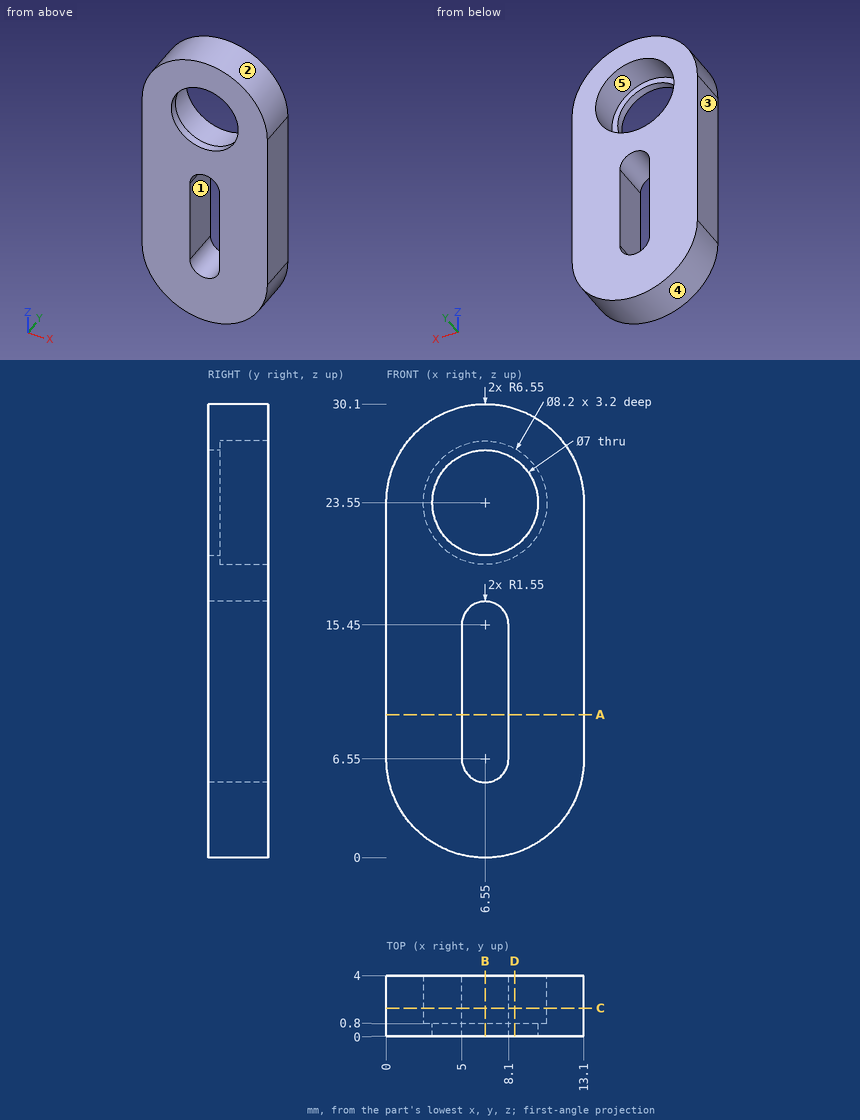
The figure shows three views and two pictorial views of one solid part (mm, origin at its lowest corner). Answer the questions. A direction names the side the tool comes from. Coordinates: 2 decimals unless noted, no trailing zeros. Loops run counter-clockwise (first coordinate to the right, second up) from the corner with the lowest first, then second, coordinate; pieces in that order, holes last. Notation, with made-up numbers: (-22, -2.75) -> (34, -2.75) arc R21 ccw to (34, 35.25) -> close; hole circle Ø3 at (15, 77.5). An arc over 180 degrees is marked (long way). Use one line per item in the form item = value. Start each with the question number.
Item 1: A tool of negligible diameter and unlimited length cuts with its end or side. For the marked faces 1 and 2, from which of +Z, -Z, +X, -X, +Y, -Y can it reach the whole face along a straight path? Write none if from no direction.
Item 2: The part is cut by section B-B on x = 6.55. Determine the outline of the cut face in (y, z), then the cut area to 3 significant figures.
Item 3: Consider L1, parallel to Z at x = 6.55, y = 2.35; L2, parallel to Z at x = 6.55, y = 0.3; L3, parallel to X at y = 3.45, z = 12.5. Determine where each line is inside the solid, lowest interval first. Write a range as [from, to].
Item 4: Flat-ended cylindrical pins translate along their axes: pin 1 Ø3 at (x, z) = (3, 9.5) entering from -Y; pin 2 Ø1 at (x, y) = (11.5, 1) entering from -Z; pin 3 Ø6.5 at (x, z) = (6.55, 23.55) entering from +Y. Find the tip coordinate at first contact, or state that the pin passes through.
Item 5: The mould has two halves that part along X. Classify the marked faces 3, 4 and 5: released by +X, released by -X, zero draft, split by the parting line, or undercut.
Item 6: The part is cut by section A-A on z = 9.5. Determine the outline of the cut face in (x, y), then the cut area to 3 significant figures.
Item 7: The part is cut by section C-C on y = 1.85. Determine the outline of the cut face in (x, z), then the cut area to 3 significant figures.
Item 8: The part is cut by section D-D on x = 8.5. Determine the outline of the cut face in (y, z), then the cut area to 3 significant figures.
Answer key:
q1.face_1 = +Y, -Y
q1.face_2 = +Z, +Y, -Y
q2.outline = (0, 0) -> (4, 0) -> (4, 5) -> (0, 5) -> close; (0, 17) -> (4, 17) -> (4, 19.45) -> (0.8, 19.45) -> (0.8, 20.05) -> (0, 20.05) -> close; (0, 27.05) -> (0.8, 27.05) -> (0.8, 27.65) -> (4, 27.65) -> (4, 30.1) -> (0, 30.1) -> close
q2.area = 40.6 mm2
q3.L1 = [0, 5], [17, 19.45], [27.65, 30.1]
q3.L2 = [0, 5], [17, 20.05], [27.05, 30.1]
q3.L3 = [0, 5], [8.1, 13.1]
q4.pin_1 = 0
q4.pin_2 = 1.74
q4.pin_3 = through
q5.face_3 = released by -X
q5.face_4 = split by the parting line
q5.face_5 = undercut
q6.outline = (0, 0) -> (5, 0) -> (5, 4) -> (0, 4) -> close; (8.1, 0) -> (13.1, 0) -> (13.1, 4) -> (8.1, 4) -> close
q6.area = 40.0 mm2
q7.outline = (0, 6.55) arc R6.55 ccw to (13.1, 6.55) -> (13.1, 23.55) arc R6.55 ccw to (0, 23.55) -> close; hole circle Ø8.2 at (6.55, 23.55); hole (5, 6.55) arc R1.55 ccw to (8.1, 6.55) -> (8.1, 15.45) arc R1.55 ccw to (5, 15.45) -> close
q7.area = 270 mm2
q8.outline = (0, 0.3) -> (4, 0.3) -> (4, 19.94) -> (0.8, 19.94) -> (0.8, 20.64) -> (0, 20.64) -> close; (0, 26.46) -> (0.8, 26.46) -> (0.8, 27.16) -> (4, 27.16) -> (4, 29.8) -> (0, 29.8) -> close
q8.area = 90.3 mm2
